Verification items for the finished model (mm, model axes). A direction names the side the tool comes from. Coordinates: 2 decimals unless noted, no trailing zeros. Loops run counter-clockwise (first coordinate to the right, second up) from the corner with the lowest first, then second, coordinate; pieces in that order, holes last. Notation, with made-up numbers: (42, -24) -> (49, -24) arc R20 cw to (49, -19) -> close; hole circle Ø11 at (9, -20.75). An arc over 180 degrees is marked (long way). Answer as a JSON object with one key per item and string values. Group by question number.
Q1. Cross-section at A-A on y = 2. Record the boundary of the cut face in (x, z).
Q2. Cross-section at C-C on x = 1.15. Record the boundary of the cut face in (y, z).
Q3. Scan lines: L1, parallel to X at y = -4.5, z = 12; L2, parallel to Z at x = -1.3, y = -0.75; L3, parallel to Y at x = 1.75, z = 2.25. Record each from-to range of solid material in increasing order.
Q4. Cross-section at D-D on x = -2.05. Record the boundary of the cut face in (y, z), and give its area (3 significant figures).
Q5. Cross-section at B-B on z = 12. Record the boundary of the cut face in (x, y), and give its area (3 significant figures).
Q6. Release check for a two-part mould opening along Z. For faces 1 (the cylindrical face through (-0.35, -4.49, 8.56)), 2 (the flat face through (3, -4.5, 5.3)), 3 (the cylindrical face through (0.042, -3.715, 1.301)), 4 (the cylindrical face through (-0.35, -4.49, 13.56)) record: released by +Z, released by -Z, zero draft, split by the parting line, or undercut.
Q7. Set-up check for faces 5 (the flat face through (0, 0, 1)), 6 (the flat face through (1, -5, 9)): record each of +Z, -Z, +X, -X, +Y, -Y from which the full face is reachable in a straight line by a thin tool's end or side.
Q8. Gauge pin test, flat ends, axial feed: pin 1 Ø1.8 at (x, z) = (1, 6) entering from +Y; pin 2 Ø1.9 at (x, z) = (0, 12) entering from -Y. Record the tip position at first contact, or that the pin passes through.
Autodesk Inventor part; units mm, degrees
ref_plane "YZ Plane" through (0, 0, 0) normal (1, 0, 0) x (0, 1, 0)
ref_plane "XZ Plane" through (0, 0, 0) normal (0, 1, 0) x (-1, 0, 0)
ref_plane "XY Plane" through (0, 0, 0) normal (0, 0, 1) x (1, 0, 0)
sketch "Sketch1" plane through (0, 0, 0) normal (0, 0, 1) x (1, 0, 0)
  line L0 (-3, 5) -> (3, 5)
  line L1 (3, 5) -> (3, -5)
  line L2 (3, -5) -> (-3, -5)
  line L3 (-3, -5) -> (-3, 5)
  line L4 (-3, 5) -> (3, -5) construction
  line L5 (3, 5) -> (-3, -5) construction
  circle A0 centre (0, 2) radius 1.6
  point P0 (0, 0)
  dimension "d0" = 10
  dimension "d1" = 6
  dimension "d3" = 3.2
  dimension "d4" = 3
extrude "Plate1" add sketch "Sketch1" along normal blind 1
sketch "Sketch2" plane through (3, -4, 0) normal (0, -1, 0) x (1, 0, 0)
  line L0 (-6, 0) -> (0, 0)
  line L1 (0, 0) -> (0, 15)
  line L2 (0, 15) -> (-6, 15)
  line L3 (-6, 15) -> (-6, 0)
edge flange "Flange1" height 15 angle 90 thickness 1 bend radius 1 thickness toward (0, -1, 0) relief tear relief width 1 relief depth 0.5 edges at (0, -5, 1) wall of the first edge with corners at (-3, -4, 0) (3, -4, 0) (3, -4, 15) (-3, -4, 15)
bend "Bend1"
corner "Corner1"
sketch "Sketch3" plane through (-3, -4, 15) normal (0, 1, 0) x (1, 0, 0)
  circle A0 centre (3, 3) radius 1.6
  circle A1 centre (3, 8) radius 1.6
  line L0 (0, 0) -> (6, 0)
  point P0 (3, 15)
  point P1 (3, 0)
  dimension "d15" = 3.2
  dimension "d16" = 3.2
  dimension "d17" = 5
  dimension "d18" = 3
extrude "Cut1" cut sketch "Sketch3" against normal blind 1
equation "\"d19\" = 厚度"
equation "\"d2\" = 厚度"
equation "\"d5\" = 折彎離隙寬度"
equation "\"d6\" = 折彎離隙深度"
equation "\"d7\" = 最小剩餘"
equation "\"d8\" = 轉移半徑"
equation "\"d11\" = 折彎半徑"
equation "\"d12\" = 轉角離隙大小"
equation "\"d13\" = 間隙大小"
equation "\"d14\" = Jacobi半徑大小"
equation "\"折彎半徑\" = 厚度"
equation "\"折彎離隙寬度\" = 厚度"
equation "\"折彎離隙深度\" = 0.5 * 厚度"
equation "\"轉角離隙大小\" = 4 * 厚度"
equation "\"最小剩餘\" = 2 * 厚度"
equation "\"轉移半徑\" = 折彎半徑"
equation "\"Jacobi半徑大小\" = 折彎半徑"
equation "\"間隙大小\" = 厚度"
properties part number "connector2_cooler"
Computed values:
{
 "1": {"outline": "(-3, 0) -> (-1.6, 0) -> (-1.6, 1) -> (-3, 1) -> close; (1.6, 0) -> (3, 0) -> (3, 1) -> (1.6, 1) -> close"},
 "2": {"outline": "(-5, 2) arc R2 ccw to (-3, 0) -> (0.89, 0) -> (0.89, 1) -> (-3, 1) arc R1 cw to (-4, 2) -> (-4, 5.89) -> (-5, 5.89) -> close; (-5, 8.11) -> (-4, 8.11) -> (-4, 10.89) -> (-5, 10.89) -> close; (-5, 13.11) -> (-4, 13.11) -> (-4, 15) -> (-5, 15) -> close; (3.11, 0) -> (5, 0) -> (5, 1) -> (3.11, 1) -> close"},
 "3": {"L1": "x = -3 to -1.6, 1.6 to 3", "L2": "z = 0 to 1", "L3": "y = -5 to -4"},
 "4": {"outline": "(-5, 2) arc R2 ccw to (-3, 0) -> (5, 0) -> (5, 1) -> (-3, 1) arc R1 cw to (-4, 2) -> (-4, 15) -> (-5, 15) -> close", "area": "23.4 mm²"},
 "5": {"outline": "(-3, -5) -> (-1.6, -5) -> (-1.6, -4) -> (-3, -4) -> close; (1.6, -5) -> (3, -5) -> (3, -4) -> (1.6, -4) -> close", "area": "2.80 mm²"},
 "6": {"face 1": "undercut", "face 2": "zero draft", "face 3": "released by +Z", "face 4": "undercut"},
 "7": {"face 5": "+Z, +X, -X, +Y", "face 6": "+Z, -Z, +X, -X, -Y"},
 "8": {"pin 1": "stops at y = -4", "pin 2": "passes through"}
}
